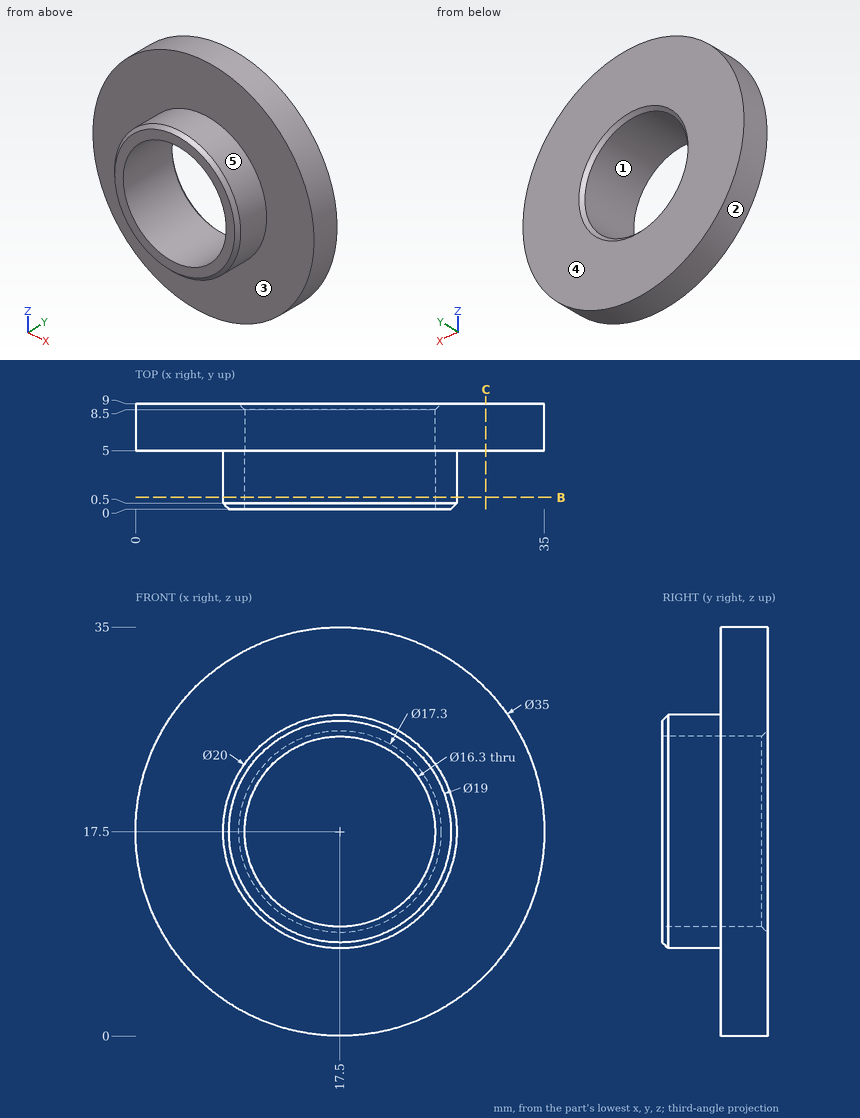
For this review, use the dimensioned drawing (mm, ordinates from the lowest corner) and the shaded views. A direction names the side the tool comes from. Coordinates: 2 decimals unless noted, no trailing zeros. Loops run counter-clockwise (first coordinate to the right, second up) from the corner with the lowest first, then second, coordinate; pieces in that order, holes last. Notation, with made-up numbers: M 47.25,72.25 L 64.25,72.25 A18 cw 64.25,80.25 Z; hole C 43.5,10.5 d10. An arc over 180 degrees is marked long. Answer as CSV lines item,"result".
Item 1: Add section B-B on y = 1. State the section outline as (x, z) points.
Answer list:
outline,"C 17.5,17.5 d20; hole C 17.5,17.5 d16.3"
Item 2: For probe 1 along Z at (x, y) = (17.5, 6.75); probe 2 along Z at (x, y) = (17.5, 4.5), list the stretches that pass through material, from the lowest coordinate up.
Answer list:
probe 1,"0 to 9.35, 25.65 to 35"
probe 2,"7.5 to 9.35, 25.65 to 27.5"
Item 3: The part is to be moulded in two halves that separate along X. For the marked faces 1, 2 and 3, say which applies: pulls with the +X half, pulls with the -X half, needs draft (parallel to the pull), parting line crosses it, or undercut.
Answer list:
face 1,"undercut"
face 2,"parting line crosses it"
face 3,"needs draft"
Item 4: For P1, Ø1.5, axis at x = 25.5, y = 2, coming from the -Z side; P2, Ø5, axis at x = 20.5, z = 20, coming from the -Y side; P3, Ø4, axis at x = 24, y = 5, coming from the -Z side; P4, Ø10, axis at x = 20.5, z = 6, coming from the -Y side, all flat-tipped, find the tip position at first contact; note any pin that passes through.
Answer list:
P1,"z = 10.61"
P2,"through"
P3,"z = 0.59"
P4,"y = 0"
Item 5: Machinability: for the marked faces 4 and 5, which of the approach directions +Z, -Z, +X, -X, +Y, -Y give a long, thin tool a straight path to every point of the face, cutting with its end or side? Answer none if there is none.
Answer list:
face 4,"+Z, -Z, +X, -X, +Y"
face 5,"-Y"
Item 6: Add section C-C on x = 30. State the section outline as (y, z) points.
Answer list:
outline,"M 5,5.25 L 9,5.25 L 9,29.75 L 5,29.75 Z"
